```python
from build123d import *

# Parameters (mm, degrees)
SKETCH1_W            = 100
SKETCH1_H            = 50
BOSS_EXTRUDE1_DEPTH  = 10
SKETCH2_R            = 5
CUT_EXTRUDE1_DEPTH   = 10
LPATTERN1_COUNT      = 5
LPATTERN1_PITCH      = 20
LPATTERN1_COUNT_DIR2 = 3
LPATTERN1_PITCH_DIR2 = 20


with BuildPart() as part:
    # Sketch1 → Boss-Extrude1 (new body)
    with BuildSketch(Plane(origin=(0, 0, 0), x_dir=(1, 0, 0), z_dir=(0, 1, 0))):
        Rectangle(SKETCH1_W, SKETCH1_H)
    extrude(amount=BOSS_EXTRUDE1_DEPTH)

    # Sketch2 → Cut-Extrude1 (cut)
    with BuildSketch(Plane(origin=(0, 10, 0), x_dir=(1, 0, 0), z_dir=(0, 1, 0))):
        with Locations(Location((-40, 15, 0), (0, 0, 270))):
            Circle(SKETCH2_R)
    cut_extrude1 = extrude(amount=-CUT_EXTRUDE1_DEPTH, mode=Mode.SUBTRACT)

    # LPattern1: Cut-Extrude1 5 × 3, 1 skipped
    with Locations(*[(i * LPATTERN1_PITCH, 0, j * LPATTERN1_PITCH_DIR2) for i in range(LPATTERN1_COUNT) for j in range(LPATTERN1_COUNT_DIR2) if (i, j) not in ((0, 0), (2, 1))]):
        add(cut_extrude1, mode=Mode.SUBTRACT)


solid = part.part
```
Here's how the part is built. I have some questions about the finished solid (model axes, mm). Give positions to 0.01 mm unless a question says otherwise; leave off trailing zeros. Loops run counter-clockwise (first coordinate to the right, second up) from the corner with the lowest first, then second, coordinate; pieces in that order, holes last. Notation, with made-up numbers: M -6,-33.5 L 26,-33.5 A21 cw 26,-27.5 Z; hole C 89,55.5 d6. An arc over 180 degrees is marked long. Use one line per item in the form item = value. Start each with the question number.
Q1. If we section it at C-C (x = -17): Write out the boundary of the cut face in (y, z), then the cut area to 3 significant figures.
Q2. I need wall thicknesses on line 1 along X through (y, z) = (6.5, 5); line 2 along X through (y, z) = (5.5, -15); line 3 along X through (y, z) = (7.75, 8). Which ranges of each line are inside material? Lowest first, please.
Q3. If we section it at B-B (x = 0): Write out the boundary of the cut face in (y, z), then the cut area to 3 significant figures.
Q4. If we section it at D-D (z = 5): Write out the boundary of the cut face in (x, y), then the cut area to 3 significant figures.
Q5. Will these pins go through, and if not, where does the flat tip stop? pin 1 Ø8 at (x, z) = (40, 5) entering from +Y; pin 2 Ø2 at (x, y) = (0, 5) entering from +Z.
Q6. Thinking about a two-plate mould opening in X: for faces 1 (the flat face through (47, 5, 25)), 2 (the cylindrical face through (-40, 5, 20)), 3 (the flat face through (-50, 5, 0)), which applies, +X half, -X half, draft (parallel to the pull), parting line (faces both ways), or undercut?
Q7. If we section it at A-A (z = -11): Write out the boundary of the cut face in (x, y).
Taken from the geometry:
q1.outline = M 0,-25 L 10,-25 L 10,-19 L 0,-19 Z; M 0,-11 L 10,-11 L 10,1 L 0,1 Z; M 0,9 L 10,9 L 10,21 L 0,21 Z
q1.area = 300 mm^2
q2.line_1 = -50 to -45, -35 to -25, -15 to 15, 25 to 35, 45 to 50
q2.line_2 = -50 to -45, -35 to -25, -15 to -5, 5 to 15, 25 to 35, 45 to 50
q2.line_3 = -50 to -44, -36 to -24, -16 to 16, 24 to 36, 44 to 50
q3.outline = M 0,-25 L 10,-25 L 10,-20 L 0,-20 Z; M 0,-10 L 10,-10 L 10,20 L 0,20 Z
q3.area = 350 mm^2
q4.outline = M -50,0 L -45,0 L -45,10 L -50,10 Z; M -35,0 L -25,0 L -25,10 L -35,10 Z; M -15,0 L 15,0 L 15,10 L -15,10 Z; M 25,0 L 35,0 L 35,10 L 25,10 Z; M 45,0 L 50,0 L 50,10 L 45,10 Z
q4.area = 600 mm^2
q5.pin_1 = through
q5.pin_2 = 20.1
q6.face_1 = draft
q6.face_2 = undercut
q6.face_3 = -X half
q7.outline = M -50,0 L -43,0 L -43,10 L -50,10 Z; M -37,0 L -23,0 L -23,10 L -37,10 Z; M -17,0 L -3,0 L -3,10 L -17,10 Z; M 3,0 L 17,0 L 17,10 L 3,10 Z; M 23,0 L 37,0 L 37,10 L 23,10 Z; M 43,0 L 50,0 L 50,10 L 43,10 Z
